from build123d import *

# Parameters (mm, degrees)
SKETCH_1_W          = 100
SKETCH_1_H          = 200
EXTRUDE_1_DEPTH     = 100
SKETCH_2_R          = 30
SKETCH_2_W          = 70
SKETCH_2_H          = 40
CUT_EXTRUDE_1_DEPTH = 101


with BuildPart() as part:
    # 草图1 → 凸台-拉伸1 (new body)
    with BuildSketch(Plane.XY):
        with Locations((-8.762886598, -29.896907216)):
            Rectangle(SKETCH_1_W, SKETCH_1_H)
    extrude(amount=EXTRUDE_1_DEPTH)

    # 草图2 → 切除-拉伸1 (cut, through all)
    with BuildSketch(Plane(origin=(41.237113402, 0, 0), x_dir=(0, 0, -1), z_dir=(1, 0, 0))):
        with Locations((-50, 30.103092784)):
            Circle(SKETCH_2_R)
        with Locations((-50, -99.896907216)):
            Rectangle(SKETCH_2_W, SKETCH_2_H)
    extrude(amount=-CUT_EXTRUDE_1_DEPTH, mode=Mode.SUBTRACT)


solid = part.part
CAD build for the part. Positions are in the model's coordinates, mm. A direction names the side the tool comes from. Coordinates: 2 decimals unless noted, no trailing zeros. Write each loop counter-clockwise with the first axis right and the second up, starting at its lowest first coordinate (ties: lowest second). Pieces come first, ordered by that corner, then holes. Notation, with made-up numbers: (66, 41.5) - (94, 41.5) arc R19 cw to (94, 61.5) - close; hole circle Ø5 at (65.25, -20.75). An arc over 180 degrees is marked (long way). Use a Markdown table: item, result. Add a question column.
Item 1: Band-saw the part on A-A, the plane z = 50. Give the cut face in (x, y), and give its area (3 significant figures).
Item 2: Drill centre lines: L1, parallel to Y at x = -25, z = 50; L2, parallel to Z at x = 32.5, y = -88; L3, parallel to Y at x = -18.5, z = 81. Where is each one in solid material? Low to high. Write a range as from..to.
Item 3: Mould opens along Z. For faces 3 (the face through (-58.763, -31, 49)), 4 (the face through (-9, -28, 100)), 5 (the face through (-8, -79.897, 50)) say: pulls with the +Z half, pulls with the -Z half, needs draft (parallel to the pull), parting line crosses it, or undercut.
Item 4: Band-saw the part on B-B, the plane y = -99.5. Give the cut face in (x, z).
Item 5: Band-saw the part on D-D, the plane z = 64. Give the cut face in (x, y), and give its area (3 significant figures).
Item 6: Band-saw the part on C-C, the plane x = 2.5. Give the cut face in (y, z), and give its area (3 significant figures).
Item 7: 3-axis set-ups, long thin cutter, end or side, ignore diameter. For faces 1 (the face through (-8, -100, 15)), 2 (the face through (-9, -28, 0)): which of +Z, -Z, +X, -X, +Y, -Y reach the whole face in a straight line?
Numbers:
| question | item | result |
|---|---|---|
| 1 | outline | (-58.76, -129.9) - (41.24, -129.9) - (41.24, -119.9) - (-58.76, -119.9) - close; (-58.76, -79.9) - (41.24, -79.9) - (41.24, 0.1) - (-58.76, 0.1) - close; (-58.76, 60.1) - (41.24, 60.1) - (41.24, 70.1) - (-58.76, 70.1) - close |
| 1 | area | 10,000 mm2 |
| 2 | L1 | -129.9..-119.9, -79.9..0.1, 60.1..70.1 |
| 2 | L2 | 0..15, 85..100 |
| 2 | L3 | -129.9..-119.9, -79.9..70.1 |
| 3 | face 3 | needs draft |
| 3 | face 4 | pulls with the +Z half |
| 3 | face 5 | undercut |
| 4 | outline | (-58.76, 0) - (41.24, 0) - (41.24, 15) - (-58.76, 15) - close; (-58.76, 85) - (41.24, 85) - (41.24, 100) - (-58.76, 100) - close |
| 5 | outline | (-58.76, -129.9) - (41.24, -129.9) - (41.24, -119.9) - (-58.76, -119.9) - close; (-58.76, -79.9) - (41.24, -79.9) - (41.24, 3.57) - (-58.76, 3.57) - close; (-58.76, 56.64) - (41.24, 56.64) - (41.24, 70.1) - (-58.76, 70.1) - close |
| 5 | area | 10,700 mm2 |
| 6 | outline | (-129.9, 0) - (70.1, 0) - (70.1, 100) - (-129.9, 100) - close; hole (-119.9, 15) - (-79.9, 15) - (-79.9, 85) - (-119.9, 85) - close; hole circle Ø60 at (30.1, 50) |
| 6 | area | 14,400 mm2 |
| 7 | face 1 | +X, -X |
| 7 | face 2 | -Z, +X, -X, +Y, -Y |
